Verification items for this drawing (mm, ordinates from the low corner). Coordinates: 2 decimals unless noted, no trailing zeros. Write each loop counter-clockwise with the first axis right and the second up, starting at its lowest first coordinate (ties: lowest second). Pieces come first, ordered by that corner, then holes. Notation, with made-up numbers: M -28,50.5 L -7,50.5 A19 cw -7,78.5 Z; hole C 69,62 d3. An arc over 180 degrees is marked long. Answer as CSV lines item,"result". Start each with the question number.
1) Material ranges on L1, parallel to Y at x = 3.5, z = 3.25; L2, parallel to X at y = 1.5, z = 9.5; L3, parallel to X at y = 1.5, z = 10.25, recorded low to high. Write a range as [from, to].
2) Go/stop test with flat-tipped pins: pin 1 Ø1.5 at (x, z) = (2, 4) entering from +Y; pin 2 Ø2 at (y, z) = (5, 8) entering from +X; pin 3 Ø2 at (y, z) = (5.5, 8.5) entering from +X. Record where each tip stops, or that it passes through.
3) Section check C-C (z = 1.25). Record the cut outline in (x, y), and give its area (3 significant figures).
4) Draft check along Y on the marked faces 1 and 2. Enter one of: +Y half, -Y half, draft (parallel to the pull), parting line (faces both ways), or undercut.
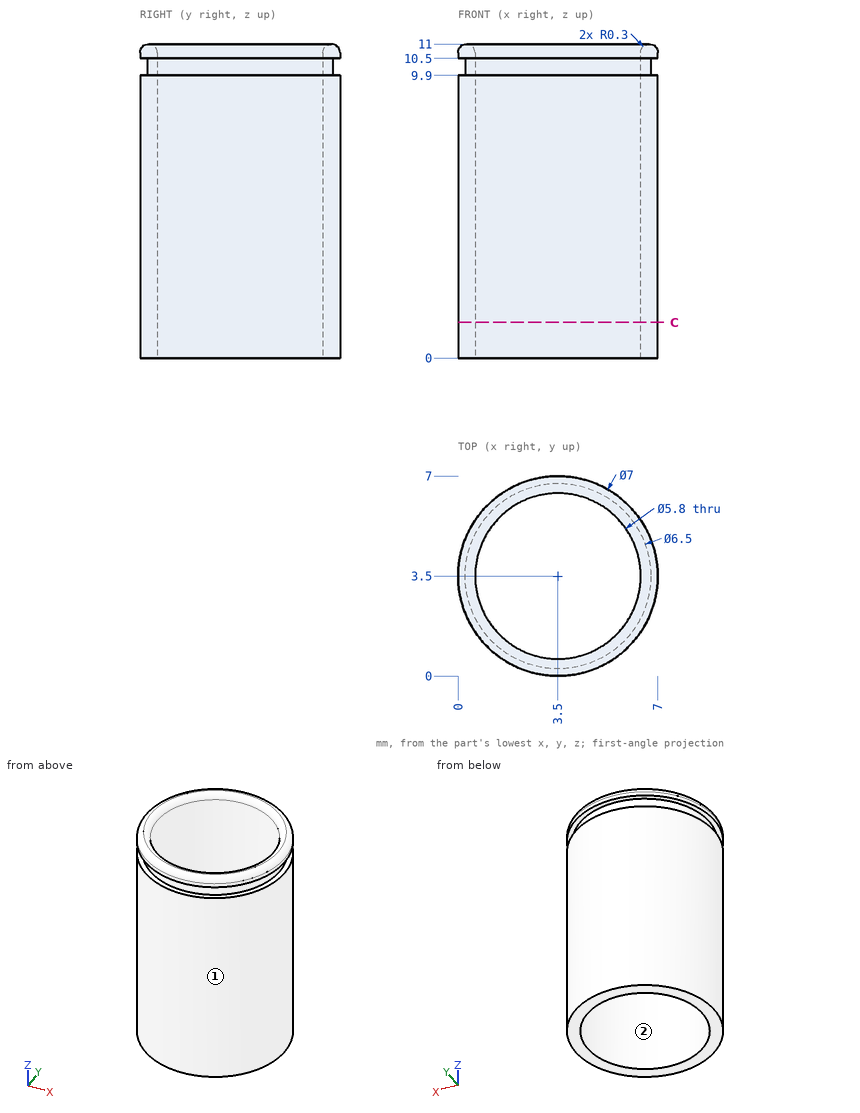
Results found:
1,L1,"y = [0, 0.6], [6.4, 7]"
1,L2,"x = [0.63, 1.4], [5.6, 6.37]"
1,L3,"x = [0.94, 1.4], [5.6, 6.06]"
2,pin 1,"stops at y = 6.92"
2,pin 2,"stops at x = 6.96"
2,pin 3,"stops at x = 6.85"
3,outline,"C 3.5,3.5 d7; hole C 3.5,3.5 d5.8"
3,area,"12.1 mm2"
4,face 1,"parting line"
4,face 2,"undercut"
